Geometry check sheet. Reference: the model listing, model coordinates, mm. Face numbers are marked on the shaded views. Give positions to 0.01 mm unless a question says otherwise; leave off trailing zeros. Loops run counter-clockwise (first coordinate to the right, second up) from the corner with the lowest first, then second, coordinate; pieces in that order, holes last. Notation, with made-up numbers: (70, 4) -> (109, 4) arc R27 ccw to (109, 38) -> close; hole circle Ø2 at (-5, 18). An arc over 180 degrees is marked (long way). One line per item, written item: value. Start each with the question number.
(1) Sectioned sample at B-B, the plane x = 0. Record the cut outline in (y, z) (3 decimals).
(2) Sectioned sample at D-D, the plane y = -5. Record the cut outline in (x, z) (3 decimals), then the cut area to 3 significant figures.
(3) Draft check along Y on the marked faces 1, 2, 3 and 4. Enter one of: pulls with the +Y half, pulls with the -Y half, needs draft (parallel to the pull), parting line crosses it, or undercut.
(4) Gauge pin test, flat ends, axial feed: pin 1 Ø2 at (y, z) = (-24.5, 13.5) entering from -X; pin 2 Ø6 at (y, z) = (-27.5, 41) entering from -X; pin 3 Ø12 at (x, y) = (-5, -55.5) entering from +Z. Record the tip position at first contact, or that the pin passes through.
(5) Sectioned sample at C-C, the plane y = -42.5. Record the cut outline in (x, z) (3 decimals).
(6) Scan lines: line 1 along Y through (x, z) = (-4, 23.5); line 2 along Z through (x, y) = (0, -5.75) (3 decimals); line 3 along Z through (x, y) = (-1.5, -12.5). Record each from-to range of solid material in increasing order. Write a range as from..to.
(7) Sectioned sample at A-A, the plane z = 0. Record the cut outline in (x, y) (3 decimals), then the cut area to 3 significant figures.
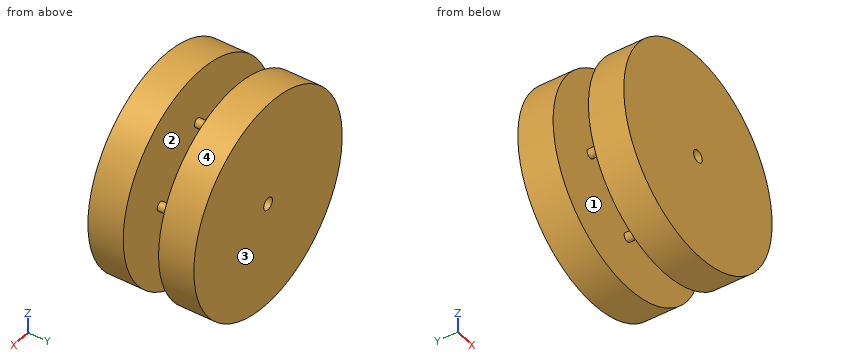
from build123d import *

# Parameters (mm, degrees)
F0_R     = 76.2
F2_DEPTH = 25.4
F1_R     = 4.445
F3_DEPTH = 25.4
F4_R     = 3.175
F5_DEPTH = 25.4
F6_R     = 76.2
F7_DEPTH = 25.4
F8_R     = 4.445
F9_DEPTH = 25.4


with BuildPart() as f2:
    # F0 (on Front) → F2 (new body)
    with BuildSketch(Plane.XZ):
        Circle(F0_R)
    extrude(amount=F2_DEPTH)

    # F1 (on face) → F3 (cut)
    with BuildSketch(Plane.XZ):
        Circle(F1_R)
    extrude(amount=F3_DEPTH, mode=Mode.SUBTRACT)

    # F4 (on face) → F5 (join)
    with BuildSketch(Plane.XZ.offset(25.4)):
        with Locations((38.1, 0)):
            Circle(F4_R)
        with Locations((0, 38.1)):
            Circle(F4_R)
        with Locations((-38.1, 0)):
            Circle(F4_R)
        with Locations((0, -38.1)):
            Circle(F4_R)
    extrude(amount=F5_DEPTH)

    # F6 (on face) → F7 (join)
    with BuildSketch(Plane.XZ.offset(50.8)):
        Circle(F6_R)
    extrude(amount=F7_DEPTH)

    # F8 (on face) → F9 (cut)
    with BuildSketch(Plane.XZ.offset(76.2)):
        Circle(F8_R)
    extrude(amount=-F9_DEPTH, mode=Mode.SUBTRACT)


solid = f2.part
Calculated:
1. outline: (-76.2, -76.2) -> (-50.8, -76.2) -> (-50.8, -41.275) -> (-25.4, -41.275) -> (-25.4, -76.2) -> (0, -76.2) -> (0, -4.445) -> (-25.4, -4.445) -> (-25.4, -34.925) -> (-50.8, -34.925) -> (-50.8, -4.445) -> (-76.2, -4.445) -> close; (-76.2, 4.445) -> (-50.8, 4.445) -> (-50.8, 34.925) -> (-25.4, 34.925) -> (-25.4, 4.445) -> (0, 4.445) -> (0, 76.2) -> (-25.4, 76.2) -> (-25.4, 41.275) -> (-50.8, 41.275) -> (-50.8, 76.2) -> (-76.2, 76.2) -> close
2. outline: circle Ø152.4 at (0, 0); hole circle Ø8.89 at (0, 0)
2. area: 18,200 mm2
3. face 1: undercut
3. face 2: undercut
3. face 3: pulls with the +Y half
3. face 4: needs draft
4. pin 1: stops at x = -75.17
4. pin 2: stops at x = -65.55
4. pin 3: stops at z = 76.2
5. outline: circle Ø6.35 at (-38.1, 0); circle Ø6.35 at (0, -38.1); circle Ø6.35 at (0, 38.1); circle Ø6.35 at (38.1, 0)
6. line 1: y = -76.2..-50.8, -25.4..0
6. line 2: z = -76.2..-4.445, 4.445..76.2
6. line 3: z = -76.19..-4.18, 4.18..76.19
7. outline: (-76.2, -76.2) -> (-4.445, -76.2) -> (-4.445, -50.8) -> (-34.925, -50.8) -> (-34.925, -25.4) -> (-4.445, -25.4) -> (-4.445, 0) -> (-76.2, 0) -> (-76.2, -25.4) -> (-41.275, -25.4) -> (-41.275, -50.8) -> (-76.2, -50.8) -> close; (4.445, -76.2) -> (76.2, -76.2) -> (76.2, -50.8) -> (41.275, -50.8) -> (41.275, -25.4) -> (76.2, -25.4) -> (76.2, 0) -> (4.445, 0) -> (4.445, -25.4) -> (34.925, -25.4) -> (34.925, -50.8) -> (4.445, -50.8) -> close
7. area: 7,610 mm2
